```python
from build123d import *

# Parameters (mm, degrees)
SKETCH1_W           = 97.79
SKETCH1_H           = 59.69
BOSS_EXTRUDE1_DEPTH = 31.75
SHELL1_T            = -2.54
SKETCH2_W           = 6.35
SKETCH2_H           = 6.35
SKETCH2_R           = 1.35
BOSS_EXTRUDE2_DEPTH = 7.62
FILLET2_R           = 0.889
BOSS_EXTRUDE3_DEPTH = 35.56
SHELL2_START        = 2.54
SHELL2_OUTLINE_W    = 33.02
SHELL2_OUTLINE_H    = 54.61
SHELL2_DEPTH        = 19.05
FILLET3_R           = 0.762


# Read off the part's stored shape, not the designer's step: Shell2
with BuildPart() as part:
    # Sketch1 → Boss-Extrude1 (new body)
    with BuildSketch(Plane(origin=(0, 0, 0), x_dir=(1, 0, 0), z_dir=(0, 1, 0))):
        Rectangle(SKETCH1_W, SKETCH1_H)
    extrude(amount=BOSS_EXTRUDE1_DEPTH)

    # Shell1
    shell1_openings = [part.faces().sort_by_distance(p)[0] for p in [
        (0, 31.75, 0),
        (48.895, 15.875, 0),
    ]]
    offset(amount=SHELL1_T, openings=shell1_openings, kind=Kind.INTERSECTION)

    # Sketch2 → Boss-Extrude2 (add)
    # profile 1 of 2: a face of its own
    with BuildSketch(Plane(origin=(0, 2.54, 0), x_dir=(1, 0, 0), z_dir=(0, 1, 0))):
        with Locations((-36.83, 0)):
            Rectangle(SKETCH2_W, SKETCH2_H)
        with Locations(Location((-36.83, 0, 0), (0, 0, 90))):
            Circle(SKETCH2_R, mode=Mode.SUBTRACT)
    # profile 2 of 2: a face of its own
    with BuildSketch(Plane(origin=(0, 2.54, 0), x_dir=(1, 0, 0), z_dir=(0, 1, 0))):
        with Locations((36.83, 0)):
            Rectangle(SKETCH2_W, SKETCH2_H)
        with Locations(Location((36.83, 0, 0), (0, 0, 90))):
            Circle(SKETCH2_R, mode=Mode.SUBTRACT)
    extrude(amount=BOSS_EXTRUDE2_DEPTH)

    # Fillet2
    fillet2_edges = [part.edges().sort_by_distance(p)[0] for p in [
        (-33.655, 2.54, 0),
        (-33.655, 6.35, 3.175),
        (-36.83, 2.54, -3.175),
        (-33.655, 6.35, -3.175),
        (-40.005, 2.54, 0),
        (-40.005, 6.35, -3.175),
        (-36.83, 2.54, 3.175),
        (-40.005, 6.35, 3.175),
        (33.655, 2.54, 0),
        (33.655, 6.35, -3.175),
        (36.83, 2.54, 3.175),
        (33.655, 6.35, 3.175),
        (40.005, 2.54, 0),
        (40.005, 6.35, 3.175),
        (36.83, 2.54, -3.175),
        (40.005, 6.35, -3.175),
    ]]
    fillet(fillet2_edges, radius=FILLET2_R)

    # Sketch4 → Boss-Extrude3 (add)
    with BuildSketch(Plane(origin=(48.895, 0, 0), x_dir=(0, 0, -1), z_dir=(1, 0, 0))):
        Polygon((-29.845, 21.59), (-27.305, 21.59), (27.305, 21.59), (29.845, 21.59), (29.845, 0), (-29.845, 0), align=None)
    extrude(amount=BOSS_EXTRUDE3_DEPTH)

    # Shell2 outline → Shell2 (cut)
    with BuildSketch(Plane(origin=(0, 0, 0), x_dir=(1, 0, 0), z_dir=(0, 1, 0)).offset(SHELL2_START)):
        with Locations((65.405, 0)):
            Rectangle(SHELL2_OUTLINE_W, SHELL2_OUTLINE_H)
    extrude(amount=SHELL2_DEPTH, mode=Mode.SUBTRACT)

    # Fillet3
    fillet3_edges = [part.edges().sort_by_distance(p)[0] for p in [
        (84.455, 10.795, 29.845),
        (84.455, 10.795, -29.845),
        (81.915, 12.065, 27.305),
        (81.915, 12.065, -27.305),
        (-46.355, 17.145, -27.305),
        (-46.355, 17.145, 27.305),
        (48.895, 26.67, 27.305),
        (48.895, 26.67, -27.305),
        (-48.895, 15.875, -29.845),
        (48.895, 26.67, -29.845),
        (48.895, 26.67, 29.845),
        (-48.895, 15.875, 29.845),
    ]]
    fillet(fillet3_edges, radius=FILLET3_R)


solid = part.part
```
Here's how the part is built. I have some questions about the finished solid (model axes, mm). A direction names the side the tool comes from. Give positions to 0.01 mm unless a question says otherwise; leave off trailing zeros. Order: outer loops, then holes, each group sorted by start corner. A loop starts at its lowest first (then second) coordinate and runs counter-clockwise, first axis right, second up. Notation, with made-up numbers: (-7.75, -0.5) -> (7.25, -0.5) arc R16 cw to (7.25, 10.5) -> close; hole circle Ø7 at (56.5, 59). An arc over 180 degrees is marked (long way). Use CSV: the item, a comma, the result in double quotes. Start each with the question number.
Item 1: Suppose I cut it at D-D (y = 25). List the corners of the cut face in (x, z) for me (3 decimals), and give its area (3 significant figures).
Item 2: Suppose I cut it at A-A (y = 8). Give the number of separate pieces and of enclosed holes in the cut face, and give its area (3 significant figures).
Item 3: Suppose I cut it at B-B (x = -14). List the corners of the cut face in (y, z) for me (3 decimals), and give its area (3 significant figures).
Item 4: Suppose I cut it at C-C (z = 20.5). List the corners of the cut face in (x, y) for me (3 decimals), and give its area (3 significant figures).
Item 5: I'm going to push flat-ended pins straight in: P1, Ø16.5, axis at x = 7, z = -4.5, coming from the +Y side; P2, Ø5, axis at x = -36, z = 1.5, coming from the +Y side; P3, Ø0.8, axis at y = 25, z = -28.5, coming from the +X side (3 decimals); P4, Ø5, axis at x = 3, z = 19, coming from the -Y side. Where does each tip first touch, or does it pass through?
Item 6: On a 3-axis mill with a long thin cutter (end or side, diameter ignored), from which of +Z, -Z, +X, -X, +Y, -Y can I reach the whole of each face in a straight line? I mean faces 3 (the flat face through (-37, 2.54, 0)), 4 (the flat face through (-15, 31.75, 29)). Say none if no direction works.
Item 7: If I drill on probe 1 along X at (y, z) = (8, 0) (3 decimals); probe 2 along Z at (x, y) = (36.83, 5.5) (3 decimals); probe 3 along X at (y, z) = (13.5, -3) (3 decimals), over which ranges is the centre line in solid material (lowest first)? Write a range as [from, to].
Item 8: Thinking about a two-plate mould opening in X: for faces 1 (the flat face through (82.4, 21.59, -0.1)), 2 (the flat face through (-40.005, 7, 0)), which applies, pulls with the +X half, pulls with the -X half, needs draft (parallel to the pull), parting line crosses it, or undercut?
Answer block:
1,outline,"(-48.895, -29.083) arc R0.762 ccw to (-48.133, -29.845) -> (48.133, -29.845) arc R0.762 ccw to (48.895, -29.083) -> (48.895, -28.067) arc R0.762 ccw to (48.133, -27.305) -> (-45.593, -27.305) arc R0.762 cw to (-46.355, -26.543) -> (-46.355, 26.543) arc R0.762 cw to (-45.593, 27.305) -> (48.133, 27.305) arc R0.762 ccw to (48.895, 28.067) -> (48.895, 29.083) arc R0.762 ccw to (48.133, 29.845) -> (-48.133, 29.845) arc R0.762 ccw to (-48.895, 29.083) -> close"
1,area,"635 mm^2"
2,separate pieces,"3"
2,enclosed holes,"3"
2,area,"1,020 mm^2"
3,outline,"(0, -29.845) -> (31.75, -29.845) -> (31.75, -27.305) -> (2.54, -27.305) -> (2.54, 27.305) -> (31.75, 27.305) -> (31.75, 29.845) -> (0, 29.845) -> close"
3,area,"300 mm^2"
4,outline,"(-48.895, 0) -> (84.455, 0) -> (84.455, 21.59) -> (81.915, 21.59) -> (81.915, 2.54) -> (-46.355, 2.54) -> (-46.355, 31.75) -> (-48.895, 31.75) -> close"
4,area,"461 mm^2"
5,P1,"stops at y = 2.54"
5,P2,"stops at y = 10.16"
5,P3,"stops at x = 48.895"
5,P4,"stops at y = 0"
6,face 3,"+Y"
6,face 4,"+Z, -Z, +X, -X, +Y"
7,probe 1,"x = [-48.895, -46.355], [-40.005, -38.18], [-35.48, -33.655], [33.655, 35.48], [38.18, 40.005], [81.915, 84.455]"
7,probe 2,"z = [-29.845, -27.305], [-3.175, -1.35], [1.35, 3.175], [27.305, 29.845]"
7,probe 3,"x = [-48.895, -46.355], [81.915, 84.455]"
8,face 1,"needs draft"
8,face 2,"undercut"
